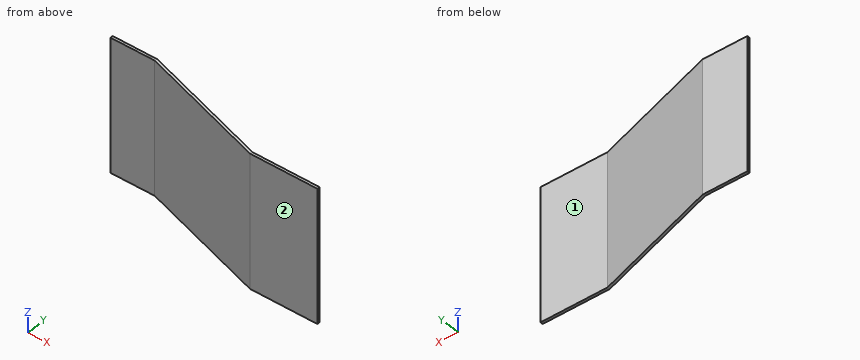
from build123d import *

# Parameters (mm, degrees)
BOSS_EXTRUDE1_DEPTH = 1000


with BuildPart() as part:
    # Sketch1 → Boss-Extrude1 (new body)
    with BuildSketch(Plane.XY):
        Polygon((0, 76.661083739), (0, 56.661083739), (338.719471809, 57.585110825), (1338.719471809, -257.414889175), (1338.719471809, -237.414889175), (1341.794983957, -237.414889175), (344.728403277, 76.661083739), align=None)
        Polygon((1338.719471809, -237.414889175), (1338.719471809, -257.414889175), (1405.287047449, -257.414889175), (1341.794983957, -237.414889175), align=None)
        Polygon((1855.588314329, -237.414889175), (1341.794983957, -237.414889175), (1405.287047449, -257.414889175), (1855.588314329, -257.414889175), align=None)
    extrude(amount=BOSS_EXTRUDE1_DEPTH)


solid = part.part
For this review, take the finished solid that the model builds, in its own axes (mm). Face numbers are marked on the shaded views. A direction names the side the tool comes from. Give positions to 0.01 mm unless a question says otherwise; leave off trailing zeros. Loops run counter-clockwise (first coordinate to the right, second up) from the corner with the lowest first, then second, coordinate; pieces in that order, holes last. Notation, with made-up numbers: M 14,-3.75 L 62,-3.75 A14 cw 62,11.25 Z; hole C 86.5,86 d6. An arc over 180 degrees is marked long. Put each result on its own line as item: value. Start each with the question number.
(1) Add section A-A, the plane z = 642. Write out the cut boundary in (x, y), then the cut area to 3 significant figures.
(2) Add section B-B, the plane x = 1662. Write out the cut boundary in (y, z).
(3) Machinability: for the marked faces 1 and 2, which of the approach directions +Z, -Z, +X, -X, +Y, -Y give a long, thin tool a straight path to every point of the face, cutting with its end or side? Answer none if there is none.
(4) For pin 1 (6 mm diameter, centred on x = 506, z = 420, fed in from -Y); pin 2 (1 mm diameter, centred on x = 445.5, z = 673.5, fed in from -Y); pin 3 (6 mm diameter, centred on x = 1551.5, z = 205.5, fed in from +Y), all flat-tipped, find the tip position at first contact; note any pin that passes through.
(5) Add section C-C, the plane y = -73.5. Write out the cut boundary in (x, z), then the cut area to 3 significant figures.
(6) Wall thickness on L1, parallel to Y at x = 1601, z = 220.5; L2, parallel to Y at x = 225, z = 467.5: over which ranges is each line inside the solid? List them lowest first.
Result:
1. outline: M 0,56.66 L 338.72,57.59 L 1338.72,-257.41 L 1855.59,-257.41 L 1855.59,-237.41 L 1341.79,-237.41 L 344.73,76.66 L 0,76.66 Z
1. area: 37,900 mm^2
2. outline: M -257.41,0 L -237.41,0 L -237.41,1000 L -257.41,1000 Z
3. face 1: +Z, -Z, +X, +Y
3. face 2: +Z, -Z, +X, -X, -Y
4. pin 1: stops at y = 3.95
4. pin 2: stops at y = 23.79
4. pin 3: stops at y = -237.41
5. outline: M 754.86,0 L 821.43,0 L 821.43,1000 L 754.86,1000 Z
5. area: 66,600 mm^2
6. L1: y = -257.41 to -237.41
6. L2: y = 57.27 to 76.66
